CAD build for the part. Positions are in the model's coordinates, mm. A direction names the side the tool comes from. Give positions to 0.01 mm unless a question says otherwise; leave off trailing zeros. Loops run counter-clockwise (first coordinate to the right, second up) from the corner with the lowest first, then second, coordinate; pieces in that order, holes last. Notation, with made-up numbers: (-21.75, 51) -> (-17.75, 51) arc R21 cw to (-17.75, 85) -> close; hole circle Ø1 at (-17, 39). An arc over 180 degrees is marked (long way). Use one line per item in the form item = value.
Solid Edge part; units mm, degrees
sketch "Sketch1" plane through (0, 0, 0) normal (0, -1, 0) x (1, 0, 0)
  line L0 (85, 75.5) -> (-85, 75.5)
  arc A0 (-100, 60.5) -> (-85, 75.5) centre (-85, 60.5) cw
  line L1 (-100, 60.5) -> (-100, 40.5)
  arc A1 (-100, 40.5) -> (-85, 25.5) centre (-85, 40.5) ccw
  line L2 (-85, 25.5) -> (85, 25.5)
  arc A2 (100, 40.5) -> (85, 25.5) centre (85, 40.5) cw
  line L3 (100, 40.5) -> (100, 60.5)
  arc A3 (85, 75.5) -> (100, 60.5) centre (85, 60.5) cw
  arc A4 (-62.5, 63.3967) -> (-61.7784, 62.0914) centre (-60.9587, 63.3967) ccw
  arc A5 (-61.7784, 62.0914) -> (-61.3341, 61.8017) centre (-70, 49) cw
  line L4 (-61.3341, 61.8017) -> (-61.3341, 61.1633)
  arc A6 (-61.3341, 61.1633) -> (-60.5164, 59.2986) centre (-58.7992, 61.1633) ccw
  arc A7 (-60.5164, 59.2986) -> (-79.7245, 59.0715) centre (-70, 49) cw
  arc A8 (-78.6659, 61.5651) -> (-79.7245, 59.0715) centre (-82.1323, 61.5651) cw
  line L5 (-78.6659, 61.8017) -> (-78.6659, 61.5651)
  arc A9 (-78.6659, 61.8017) -> (-78.5124, 61.9043) centre (-70, 49) cw
  arc A10 (-77.5, 63.7849) -> (-78.5124, 61.9043) centre (-79.7529, 63.7849) cw
  line L6 (-77.5, 66) -> (-77.5, 63.7849)
  line L7 (-69.9997, 66) -> (-77.5, 66)
  line L8 (-62.5, 66) -> (-69.9997, 66)
  line L9 (-62.5, 66) -> (-62.5, 63.3967)
  arc A11 (78.6659, 61.322) -> (79.581, 59.208) centre (81.5651, 61.322) ccw
  arc A12 (79.581, 59.208) -> (60.6967, 59.4617) centre (70, 49) cw
  arc A13 (61.3341, 60.8816) -> (60.6967, 59.4617) centre (59.434, 60.8816) cw
  line L10 (61.3341, 61.8017) -> (61.3341, 60.8816)
  arc A14 (61.3341, 61.8017) -> (61.4312, 61.8669) centre (70, 49) cw
  arc A15 (62.5, 63.8627) -> (61.4312, 61.8669) centre (60.1021, 63.8627) cw
  line L11 (62.5, 66) -> (62.5, 63.8627)
  line L12 (70, 66) -> (62.5, 66)
  line L13 (77.5, 66) -> (70, 66)
  line L14 (77.5, 66) -> (77.5, 63.4378)
  arc A16 (77.5, 63.4378) -> (78.2532, 62.0716) centre (79.1158, 63.4378) ccw
  arc A17 (78.2532, 62.0716) -> (78.6659, 61.8017) centre (70, 49) cw
  line L15 (78.6659, 61.8017) -> (78.6659, 61.322)
  line L16 (35, 48) -> (35, 53)
  line L17 (35, 53) -> (25, 53)
  line L18 (25, 53) -> (25, 48)
  line L19 (25, 48) -> (35, 48)
  line L20 (-5, 48) -> (5, 48)
  line L21 (5, 48) -> (5, 53)
  line L22 (5, 53) -> (-5, 53)
  line L23 (-5, 53) -> (-5, 48)
  line L24 (-25, 48) -> (-25, 53)
  line L25 (-25, 53) -> (-35, 53)
  line L26 (-35, 53) -> (-35, 48)
  line L27 (-35, 48) -> (-25, 48)
extrude "Protrusion1" add sketch "Sketch1" along normal blind 5
sketch "Sketch2" plane through (0, -5, 50.5) normal (0, -1, 0) x (1, 0, 0)
  line L0 (0.75, -25) -> (0.75, -11)
  line L1 (0.75, -11) -> (-0.75, -11)
  line L2 (-0.75, -11) -> (-0.75, -25)
  line L3 (0.75, -25) -> (-0.75, -25)
extrude "Cutout1" cut sketch "Sketch2" against normal blind 19.8295
1. Cut at B-B, the plane z = 44. Write the cut outline in (x, y), then the cut area to 3 significant figures.
Result sheet:
outline = (-100, -5) -> (-83.08, -5) -> (-83.08, 0) -> (-100, 0) -> close; (-56.92, -5) -> (56.92, -5) -> (56.92, 0) -> (-56.92, 0) -> close; (83.08, -5) -> (100, -5) -> (100, 0) -> (83.08, 0) -> close
area = 738 mm^2
2. Drill centre lines: line 1 (X direction, y = -3.9, z = 49); line 2 (Z direction, x = -70, y = -1.95); line 3 (X direction, y = -4.5, z = 63). Where is each one in solid material? Low to high.
Result sheet:
line_1 = -100 to -84, -56 to -35, -25 to -5, 5 to 25, 35 to 56, 84 to 100
line_2 = 25.5 to 35, 66 to 75.5
line_3 = -99.79 to -77.64, -62.45 to 62.34, 77.56 to 99.79
3. Cut at A-A, the plane x = -27.5. Write the cut outline in (y, z), then the cut area to 3 significant figures.
Result sheet:
outline = (-5, 25.5) -> (0, 25.5) -> (0, 48) -> (-5, 48) -> close; (-5, 53) -> (0, 53) -> (0, 75.5) -> (-5, 75.5) -> close
area = 225 mm^2
4. Mould opens along Z. For faces 1 (the cylindrical face through (-95.72, -2.46, 70.99)), 2 (the flat face through (1, 0, 56)), 3 (the flat face through (70, -2, 66)) say: pulls with the +Z half, pulls with the -Z half, needs draft (parallel to the pull), parting line crosses it, or undercut.
Result sheet:
face_1 = pulls with the +Z half
face_2 = needs draft
face_3 = undercut
5. Drop flat-ended pins along their axis: P1, Ø3, axis at y = -3.5, z = 64.5, coming from the -X side; P2, Ø2, axis at y = -3.5, z = 64.5, coming from the -X side; P3, Ø1.1, axis at y = -3.5, z = 64.5, coming from the +X side. Give the stop position or say it passes through.
Result sheet:
P1 = -99.79
P2 = -99.7
P3 = 99.6
6. Cut at D-D, the plane y = -2.5. State how many separate pieces and enclosed holes the cut face has, then the cut area to 3 significant figures.
Result sheet:
separate_pieces = 1
enclosed_holes = 5
area = 8,280 mm^2
7. Tool access for faces 4 (the flat face through (-0.75, -3, 33)), 5 (the flat face through (-43, -2, 25.5)), 6 (the flat face through (-30, -2, 53)): list every direction of +Z, -Z, +X, -X, +Y, -Y with a clear straight run to the whole face (end or side of a thin tool).
Result sheet:
face_4 = -Z, +Y, -Y
face_5 = -Z, +X, -X, +Y, -Y
face_6 = +Y, -Y
8. Cut at C-C, the plane x = -71. Write the cut outline in (y, z), then the cut area to 3 significant figures.
Result sheet:
outline = (-5, 25.5) -> (0, 25.5) -> (0, 35.04) -> (-5, 35.04) -> close; (-5, 66) -> (0, 66) -> (0, 75.5) -> (-5, 75.5) -> close
area = 95.2 mm^2
